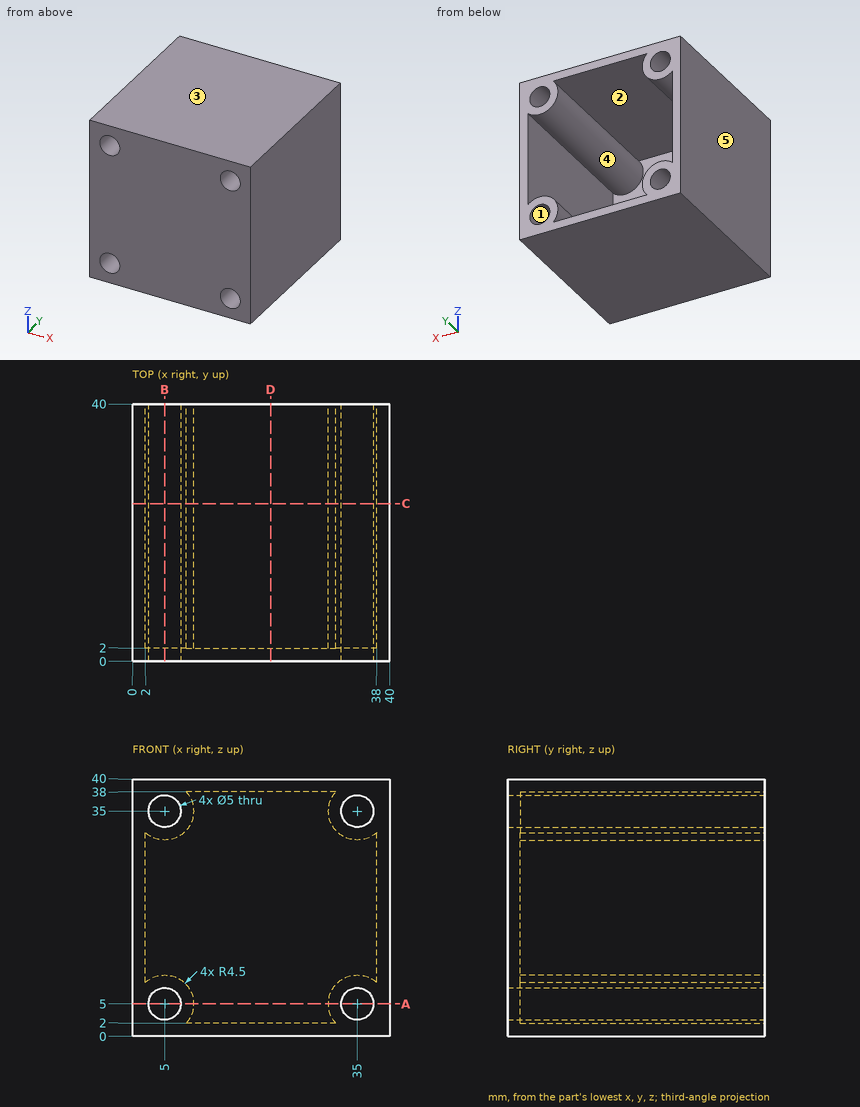
Design review of the part shown in the three views and the two pictorial views. Dimensions are in mm from the part's minimum x, y and z. A direction names the side the tool comes from. Round coordinates to 2 decimals unless told otherwise and drop trailing zeros. Loops run counter-clockwise (first coordinate to the right, second up) from the corner with the lowest first, then second, coordinate; pieces in that order, holes last. Notation, with made-up numbers: (2.25, -31) -> (6.25, -31) arc R30 ccw to (6.25, 8) -> close; hole circle Ø10 at (56, 46.25). An arc over 180 degrees is marked (long way). Answer as a JSON object with one key per item and string values. Group by question number.
1) We need section B-B on x = 5. Write out the cut boundary in (y, z), then the cut area to 3 significant figures.
2) For the marked faces 1 and 2, list the 3-axis set-ups (+Z, -Z, +X, -X, +Y, -Y) from which the entire face can be reached by the end or side of a thin tool; tool diameter is ignored.
3) For line 1 (X direction, y = 9.5, z = 35); line 2 (Z direction, x = 11.5, y = 4.5), list the stretches that pass through material, from the lowest coordinate up. Write a range as [from, to].
4) We need section C-C on y = 24.5. Write out the cut boundary in (x, z), then the cut area to 3 significant figures.
5) Mouldability with a two-part tool opening along Z and no side actions: class the marked faces 3, 4 and 5 as released by +Z, released by -Z, zero draft, split by the parting line, or undercut.
6) We need section A-A on z = 5. Write out the cut boundary in (x, y), then the cut area to 3 significant figures.
7) We need section D-D on x = 21.5. Write out the cut boundary in (y, z).
8) For pin 1 Ø5 at (x, z) = (24.5, 12.5) entering from +Y, flat-tipped, find the tip position at first contact; note if it passes through.
Result set:
{
 "1": {"outline": "(0, 0) -> (40, 0) -> (40, 2.5) -> (0, 2.5) -> close; (0, 7.5) -> (40, 7.5) -> (40, 9.5) -> (2, 9.5) -> (2, 30.5) -> (40, 30.5) -> (40, 32.5) -> (0, 32.5) -> close; (0, 37.5) -> (40, 37.5) -> (40, 40) -> (0, 40) -> close", "area": "402 mm²"},
 "2": {"face 1": "+Y, -Y", "face 2": "+Y"},
 "3": {"line 1": "[0, 2.5], [7.5, 9.5], [30.5, 32.5], [37.5, 40]", "line 2": "[0, 2], [38, 40]"},
 "4": {"outline": "(0, 0) -> (40, 0) -> (40, 40) -> (0, 40) -> close; hole (2, 8.35) arc R4.5 cw to (8.35, 2) -> (31.65, 2) arc R4.5 cw to (38, 8.35) -> (38, 31.65) arc R4.5 cw to (31.65, 38) -> (8.35, 38) arc R4.5 cw to (2, 31.65) -> close; hole circle Ø5 at (5, 5); hole circle Ø5 at (5, 35); hole circle Ø5 at (35, 5); hole circle Ø5 at (35, 35)", "area": "424 mm²"},
 "5": {"face 3": "released by +Z", "face 4": "undercut", "face 5": "zero draft"},
 "6": {"outline": "(0, 0) -> (2.5, 0) -> (2.5, 40) -> (0, 40) -> close; (7.5, 0) -> (32.5, 0) -> (32.5, 40) -> (30.5, 40) -> (30.5, 2) -> (9.5, 2) -> (9.5, 40) -> (7.5, 40) -> close; (37.5, 0) -> (40, 0) -> (40, 40) -> (37.5, 40) -> close", "area": "402 mm²"},
 "7": {"outline": "(0, 0) -> (40, 0) -> (40, 2) -> (2, 2) -> (2, 38) -> (40, 38) -> (40, 40) -> (0, 40) -> close"},
 "8": {"pin 1": "y = 2"}
}
